Print and shaded views of the part. All mm, measured from the part's lowest x, y and z. A direction names the side the tool comes from. Round coordinates to 2 decimals unless told otherwise and drop trailing zeros. Write each loop counter-clockwise with the first axis right and the second up, starting at its lowest first coordinate (ties: lowest second). Pieces come first, ordered by that corner, then holes. Notation, with made-up numbers: M 26,84.5 L 58,84.5 A19 cw 58,94.5 Z; hole C 45.25,19.25 d8. An arc over 180 degrees is marked long. Write item = value, one per line.
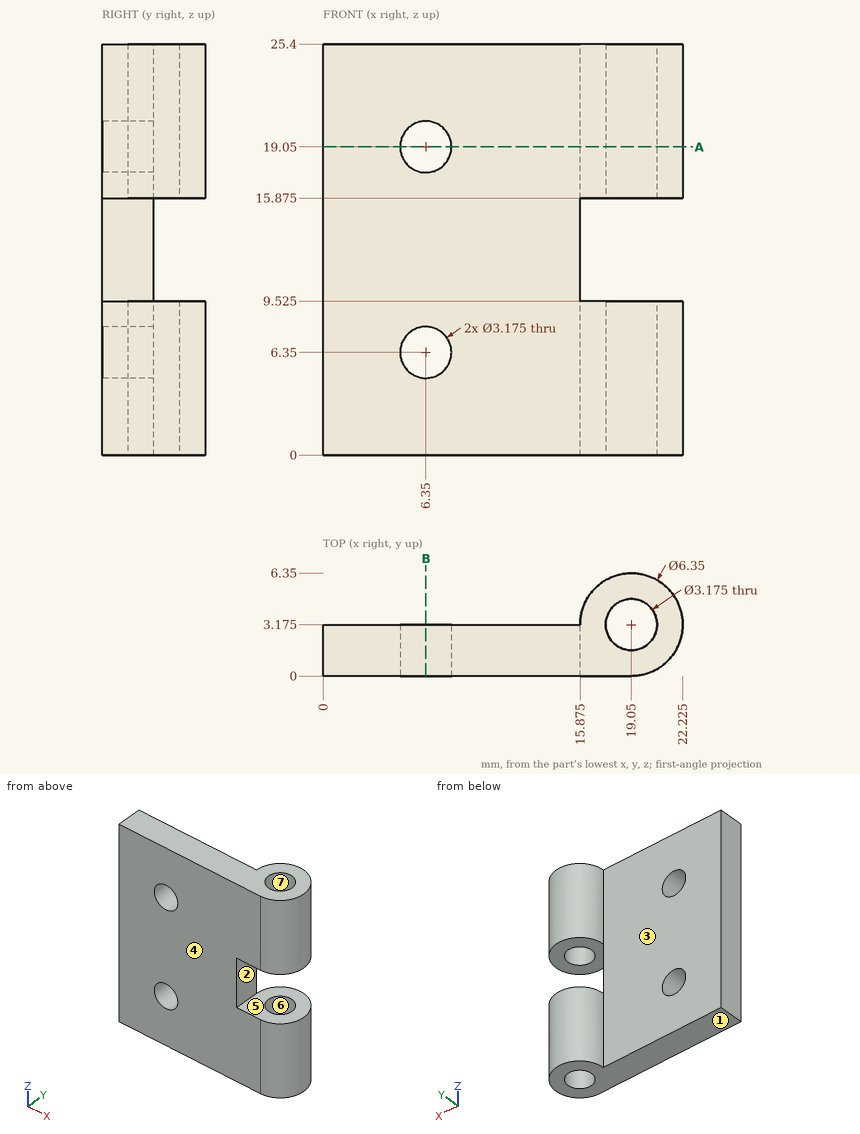
1. Band-saw the part on A-A (z = 19.05). Count the separate pieces of the cut face and the enclosed holes in it, plus the area to 3 significant figures.
Responses:
separate_pieces = 2
enclosed_holes = 1
area = 66.2 mm²
2. Mould opens along Y. For the marked faces 4, 5, 6 and 7 say: pulls with the +Y half, pulls with the -Y half, needs draft (parallel to the pull), parting line crosses it, or undercut.
Responses:
face_4 = pulls with the -Y half
face_5 = needs draft
face_6 = undercut
face_7 = undercut
3. Tool access for the marked faces 1, 2 and 3: list every direction of +Z, -Z, +X, -X, +Y, -Y with a clear straight run to the whole face (end or side of a thin tool).
Responses:
face_1 = -Z, +X, -X, +Y, -Y
face_2 = +X, +Y, -Y
face_3 = +Z, -Z, -X, +Y
4. Flat gauge pins, fed straight in: pin 1 (8 mm diameter, centred on x = 10, z = 13, fed in from +Y) (3 decimals); pin 2 (1.6 mm diameter, centred on y = 1, z = 12.5, fed in from +X) (3 decimals). Where does each tip first touch, or does it go through?
Responses:
pin_1 = 3.175
pin_2 = 15.875
5. Band-saw the part on B-B (x = 6.35). List the corners of the cut face in (y, z) (1 decimal), plus the area to 3 significant figures.
Responses:
outline = M 0,0 L 3.2,0 L 3.2,4.8 L 0,4.8 Z; M 0,7.9 L 3.2,7.9 L 3.2,17.5 L 0,17.5 Z; M 0,20.6 L 3.2,20.6 L 3.2,25.4 L 0,25.4 Z
area = 60.5 mm²
6. Probe probe 1 along Z at (x, y) = (6.25, 2); probe 2 along Y at (x, z) = (19.05, 19); probe 3 along X at (y, z) = (4.5, 4.5). List the from-to ranges inside material, lowest first.
Responses:
probe_1 = 0 to 4.77, 7.93 to 17.47, 20.63 to 25.4
probe_2 = 0 to 1.59, 4.76 to 6.35
probe_3 = 16.16 to 18.18, 19.92 to 21.94
